from build123d import *

# Parameters (mm, degrees)
BOSS_EXTRUDE1_DEPTH     = 30
CUT_EXTRUDE1_DEPTH      = 20
CUT_EXTRUDE1_DEPTH_BACK = 7
CUT_EXTRUDE3_START      = -0.5
CUT_EXTRUDE3_DEPTH      = 29
SKETCH4_R               = 0.4
CUT_EXTRUDE4_DEPTH      = 33


with BuildPart() as part:
    # Sketch1 → Boss-Extrude1 (new body)
    with BuildSketch(Plane.XY):
        with BuildLine():
            Line((-2.1, 1.334816112), (2.1, 1.334816112))
            ThreePointArc((2.1, 1.334816112), (2.948528137, 0.98334425), (3.3, 0.134816112))
            Line((3.3, 0.134816112), (3.3, -3.665183888))
            Line((3.3, -3.665183888), (-3.3, -3.665183888))
            Line((-3.3, -3.665183888), (-3.3, 0.134816112))
            ThreePointArc((-3.3, 0.134816112), (-2.948528137, 0.98334425), (-2.1, 1.334816112))
        make_face()
    extrude(amount=BOSS_EXTRUDE1_DEPTH)

    # Sketch2 → Cut-Extrude1 (cut, two sides: drawn at the far end of the back side and taken through both)
    with BuildSketch(Plane(origin=(0, 0, 0), x_dir=(0, 0, -1), z_dir=(1, 0, 0)).offset(-CUT_EXTRUDE1_DEPTH_BACK)):
        with BuildLine():
            Line((-2, 1.334816112), (-2, -0.865183888))
            Line((-2, -0.865183888), (-12, -0.865183888))
            Line((-12, -0.865183888), (-12, 0.334816112))
            ThreePointArc((-12, 0.334816112), (-12.292893219, 1.041922893), (-13, 1.334816112))
            Line((-13, 1.334816112), (-2, 1.334816112))
        make_face()
        with BuildLine():
            Line((-17, 1.334816112), (-28, 1.334816112))
            Line((-28, 1.334816112), (-28, -0.865183888))
            Line((-28, -0.865183888), (-18, -0.865183888))
            Line((-18, -0.865183888), (-18, 0.334816112))
            ThreePointArc((-18, 0.334816112), (-17.707106781, 1.041922893), (-17, 1.334816112))
        make_face()
    extrude(amount=CUT_EXTRUDE1_DEPTH + CUT_EXTRUDE1_DEPTH_BACK, mode=Mode.SUBTRACT)

    # Sketch3 → Cut-Extrude3 (cut)
    with BuildSketch(Plane(origin=(0, 0, 0), x_dir=(-1, 0, 0), z_dir=(0, 0, -1)).offset(CUT_EXTRUDE3_START)):
        with BuildLine():
            Line((-2.789484842, -3.082504219), (2.789484842, -3.082504219))
            Line((2.789484842, -3.082504219), (2.789484842, -0.711081704))
            add(Edge.make_bspline(
                [(2.789484842, -0.711081704), (2.547062941, 0.37267851), (1.996608014, 1.334816112)],
                knots=[0, 0, 0, 1, 1, 1], degree=2))
            Line((1.996608014, 1.334816112), (-1.996608014, 1.334816112))
            add(Edge.make_bspline(
                [(-2.789484842, -0.711081704), (-2.547062941, 0.37267851), (-1.996608014, 1.334816112)],
                knots=[0, 0, 0, 1, 1, 1], degree=2))
            Line((-2.789484842, -0.711081704), (-2.789484842, -3.082504219))
        make_face()
    extrude(amount=-CUT_EXTRUDE3_DEPTH, mode=Mode.SUBTRACT)

    # Sketch4 → Cut-Extrude4 (cut)
    with BuildSketch(Plane(origin=(0, 0, 0), x_dir=(-1, 0, 0), z_dir=(0, 0, -1))):
        with Locations((0, -0.646209964)):
            Circle(SKETCH4_R)
    extrude(amount=-CUT_EXTRUDE4_DEPTH, mode=Mode.SUBTRACT)


solid = part.part
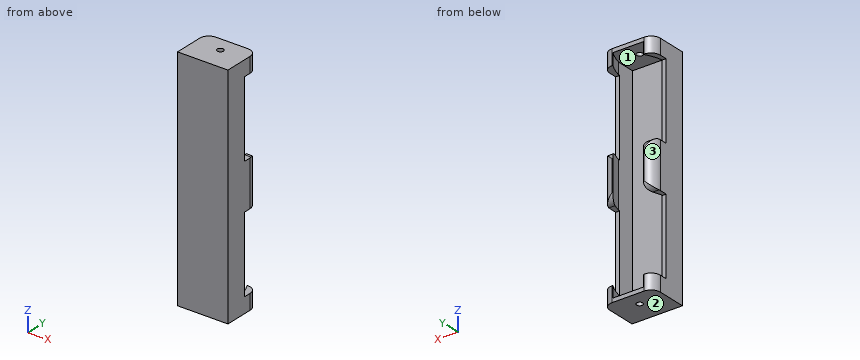
CAD build for the part. Positions are in the model's coordinates, mm. Face numbers are marked on the shaded views. Coordinates: 2 decimals unless noted, no trailing zeros. Order: outer loops, then holes, each group sorted by start corner. A loop starts at its lowest first (then second) coordinate and runs counter-clockwise, first axis right, second up.
Item 1: Band-saw the part on B-B on z = 4.5. List the corners of the cut face in (x, y), plus the area to 3 significant figures.
Check sheet entries:
outline: (-3.3, -3.67) - (3.3, -3.67) - (3.3, -0.87) - (2.79, -0.87) - (2.79, -3.08) - (-2.79, -3.08) - (-2.79, -0.87) - (-3.3, -0.87) - close
area: 6.11 mm2
Item 2: Band-saw the part on A-A on x = 0. List the corners of the cut face in (y, z), plus the area to 3 significant figures.
Check sheet entries:
outline: (-3.67, 0) - (-1.05, 0) - (-1.05, 0.5) - (-3.08, 0.5) - (-3.08, 29.5) - (-1.05, 29.5) - (-1.05, 30) - (-3.67, 30) - close; (-0.25, 0) - (1.33, 0) - (1.33, 0.5) - (-0.25, 0.5) - close; (-0.25, 29.5) - (1.33, 29.5) - (1.33, 30) - (-0.25, 30) - close
area: 21.1 mm2
Item 3: Pin check, flat tip, straight feed: pin 1 Ø1.5 at (x, z) = (-1, 10) entering from +Y. Stop position of the tip, or through.
Check sheet entries:
pin 1: stops at y = -3.08
Item 4: Two-plate mould, pull along X, no slides. Class the marked faces 1, 2 and 3: +X half, -X half, draft (parallel to the pull), parting line (faces both ways), or undercut.
Check sheet entries:
face 1: undercut
face 2: draft
face 3: -X half
Item 5: Drill centre lines: L1, parallel to Y at x = 0, z = 29.95; L2, parallel to X at y = -2.4, z = 20; L3, parallel to Z at x = -0.5, y = -0.25. Where is each one in solid material? Low to high.
Check sheet entries:
L1: y = -3.67 to -1.05, -0.25 to 1.33
L2: x = -3.3 to -2.79, 2.79 to 3.3
L3: z = 0 to 0.5, 29.5 to 30
